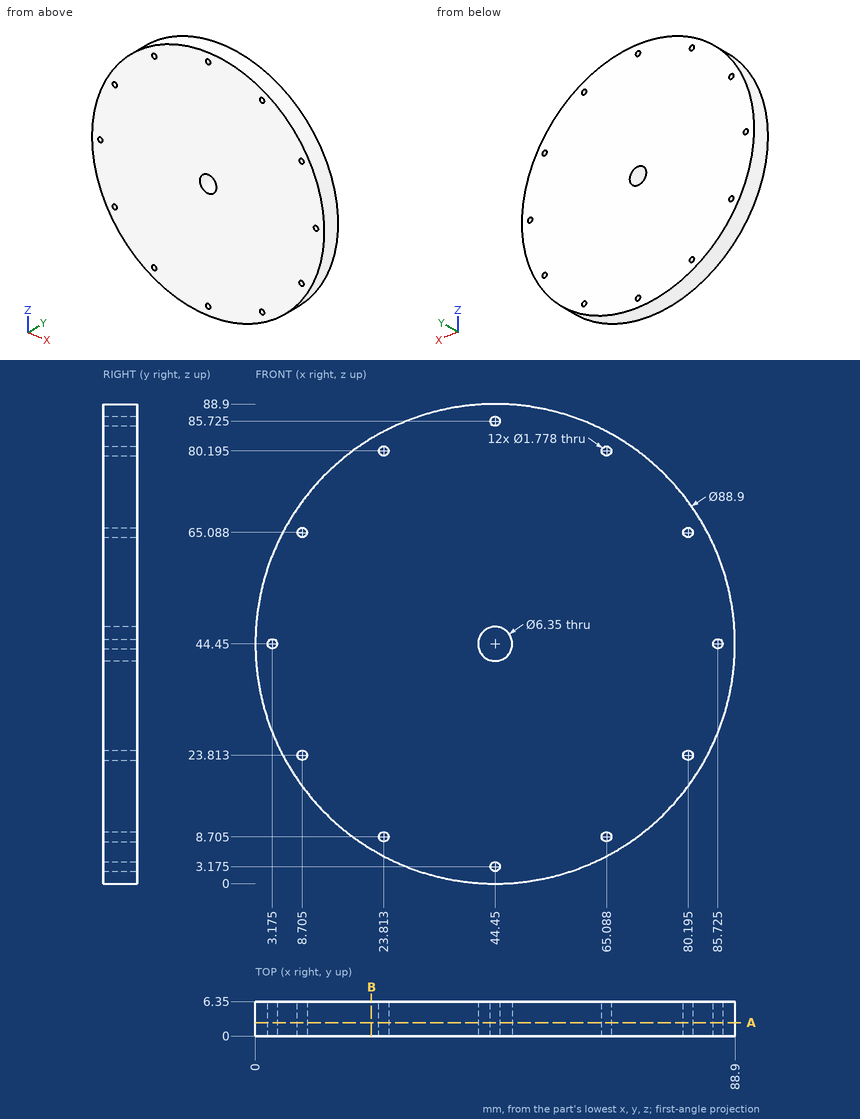
Source: three-view drawing plus pictorial views. Frame: mm from the lowest corner of the part. Coordinates: 2 decimals unless noted, no trailing zeros. Write each loop counter-clockwise with the first axis right and the second up, starting at its lowest first coordinate (ties: lowest second). Pieces come first, ordered by that corner, then holes. Notation, with made-up numbers: (-7.5, -15.75) - (2.5, -15.75) arc R19 ccw to (2.5, -11.75) - close; hole circle Ø11 at (-22, 38). An arc over 180 degrees is marked (long way). Return JSON: item names as keys, results as strings.
Item 1: Pin query (flat end, axial travel): pin 1 Ø2.5 at (x, z) = (44.45, 85.725) entering from +Y; pin 2 Ø1 at (y, z) = (3.5, 47) entering from +X; pin 3 Ø3 at (x, y) = (38.5, 1) entering from -Z. Return the tip coordinate at first contact, or that it passes through.
Completed:
{"pin 1": "stops at y = 6.35", "pin 2": "stops at x = 88.85", "pin 3": "stops at z = 0.22"}
Item 2: Line query: L1, parallel to X at y = 1.5, z = 44.45 (1 decimal); L2, parallel to X at y = 3.5, z = 23.5 (1 decimal); L3, parallel to X at y = 2.5, z = 9.5 (1 decimal). Output: solid intervals per line, ascending.
Completed:
{"L1": "x = 0 to 2.3, 4.1 to 41.3, 47.6 to 84.8, 86.6 to 88.9", "L2": "x = 5.2 to 7.9, 9.5 to 79.4, 81 to 83.7", "L3": "x = 17 to 23.4, 24.2 to 64.7, 65.5 to 71.9"}
Item 3: Section query A-A (y = 2.5). Count the separate pieces of the cut face and the enclosed holes in it, and give its area (3 significant figures).
Completed:
{"separate pieces": "1", "enclosed holes": "13", "area": "6,150 mm2"}
Item 4: Section query B-B (x = 21.5). Output: boundary loops of the cut face in (y, z).
Completed:
{"outline": "(0, 6.38) - (6.35, 6.38) - (6.35, 82.52) - (0, 82.52) - close"}
